Model file for the job. Use its own axes, mm. A direction names the side the tool comes from. Give positions to 0.01 mm unless a question says otherwise; leave off trailing zeros. Loops run counter-clockwise (first coordinate to the right, second up) from the corner with the lowest first, then second, coordinate; pieces in that order, holes last. Notation, with made-up numbers: (45.25, 70) - (67.25, 70) arc R15 cw to (67.25, 97) - close; hole circle Ø2 at (48, 56.25). An arc over 180 degrees is marked (long way). Answer as CSV lines item,"result". Start each with the question number.
Item 1: Drill centre lines: L1, parallel to Y at x = 5.5, z = 10.75; L2, parallel to Y at x = -53.45, z = 8.5; L3, parallel to X at y = -7, z = 13.5. Where is each one in solid material? Low to high. Write a range as from..to.
Item 2: Pull direction Z, two halves, no side cores. Call faces 1 (the flat face through (54, -5, 8)), 2 (the flat face through (-1, 5, 2.5)), 3 (the flat face through (-1, 12, 0)): pulls with the +Z half, pulls with the -Z half, needs draft (parallel to the pull), parting line crosses it, or undercut.
Item 3: Saw through at B-B on x = -45. Give the cut face in (y, z), plus the area to 3 significant figures.
Item 4: Saw through at A-A on y = -5. Give the cut face in (x, z).
Item 5: Tool access for faces 4 (the flat face through (39, 29.41, 1)), 5 (the cylindrical face through (54.014, 3.6, 10.325)), 6 (the flat face through (-1, -5, 2.5)), 7 (the flat face through (-39, 29.41, 1)), 8 (the cylindrical face through (53.493, -6.4, 6.675)): list every direction of +Z, -Z, +X, -X, +Y, -Y with a clear straight run to the whole face (end or side of a thin tool).
Item 6: Pin check, flat tips, straight feed: pin 1 (6 mm diameter, centred on x = 8, z = 9.5, fed in from -Y); pin 2 (1.5 mm diameter, centred on y = 11.5, z = 8.5, fed in from +X); pin 3 (4 mm diameter, centred on y = -5, z = 8.5, fed in from -X). Stop position of each tip, or through.
Item 7: Saw through at D-D on y = 32. Give the cut face in (x, z).
Item 8: Saw through at C-C on z = 13. Give the cut face in (x, y).
from build123d import *

# Parameters (mm, degrees)
SKETCH1_W           = 150
SKETCH1_H           = 41.41
BOSS_EXTRUDE1_DEPTH = 2.5
SKETCH5_W           = 110
SKETCH5_H           = 22
BOSS_EXTRUDE3_DEPTH = 12
SKETCH6_W           = 106
SKETCH6_H           = 8
CUT_EXTRUDE3_DEPTH  = 12
SKETCH7_R           = 2.3
CUT_EXTRUDE4_DEPTH  = 109
SKETCH8_R           = 2.3
CUT_EXTRUDE5_DEPTH  = 109
SKETCH9_W           = 7.040043687
SKETCH9_H           = 2.5
BOSS_EXTRUDE4_DEPTH = 20


with BuildPart() as part:
    # Sketch1 → Boss-Extrude1 (new body)
    with BuildSketch(Plane.XY):
        with Locations((0, 8.705)):
            Rectangle(SKETCH1_W, SKETCH1_H)
    extrude(amount=BOSS_EXTRUDE1_DEPTH)

    # Sketch5 → Boss-Extrude3 (add)
    with BuildSketch(Plane.XY.offset(2.5)):
        Rectangle(SKETCH5_W, SKETCH5_H)
    extrude(amount=BOSS_EXTRUDE3_DEPTH)

    # Sketch6 → Cut-Extrude3 (cut)
    with BuildSketch(Plane.XY.offset(2.5)):
        with Locations((0, 5)):
            Rectangle(SKETCH6_W, SKETCH6_H)
        with Locations((0, -5)):
            Rectangle(SKETCH6_W, SKETCH6_H)
    extrude(amount=CUT_EXTRUDE3_DEPTH, mode=Mode.SUBTRACT)

    # Sketch7 → Cut-Extrude4 (cut)
    with BuildSketch(Plane.ZY.offset(55)):
        with Locations((8.5, -5)):
            Circle(SKETCH7_R)
    extrude(amount=-CUT_EXTRUDE4_DEPTH, mode=Mode.SUBTRACT)

    # Sketch8 → Cut-Extrude5 (cut)
    with BuildSketch(Plane(origin=(55, 0, 0), x_dir=(0, 0, -1), z_dir=(1, 0, 0))):
        with Locations((-8.5, 5)):
            Circle(SKETCH8_R)
    extrude(amount=-CUT_EXTRUDE5_DEPTH, mode=Mode.SUBTRACT)

    # Sketch9 → Boss-Extrude4 (add)
    with BuildSketch(Plane(origin=(0, 29.41, 0), x_dir=(1, 0, 0), z_dir=(0, 1, 0))):
        with Locations((0.645201015, -1.25)):
            Rectangle(SKETCH9_W, SKETCH9_H)
    extrude(amount=BOSS_EXTRUDE4_DEPTH)


solid = part.part
Responses:
1,L1,"-11..-9, -1..1, 9..11"
1,L2,"-11..-7.3, -2.7..2.7, 7.3..11"
1,L3,"-55..-53, 53..55"
2,face 1,"undercut"
2,face 2,"pulls with the +Z half"
2,face 3,"pulls with the -Z half"
3,outline,"(-12, 0) - (29.41, 0) - (29.41, 2.5) - (11, 2.5) - (11, 14.5) - (9, 14.5) - (9, 2.5) - (1, 2.5) - (1, 14.5) - (-1, 14.5) - (-1, 2.5) - (-9, 2.5) - (-9, 14.5) - (-11, 14.5) - (-11, 2.5) - (-12, 2.5) - close"
3,area,"176 mm2"
4,outline,"(-75, 0) - (75, 0) - (75, 2.5) - (55, 2.5) - (55, 14.5) - (53, 14.5) - (53, 10.8) - (54, 10.8) - (54, 6.2) - (53, 6.2) - (53, 2.5) - (-53, 2.5) - (-53, 6.2) - (-55, 6.2) - (-55, 2.5) - (-75, 2.5) - close; (-55, 10.8) - (-53, 10.8) - (-53, 14.5) - (-55, 14.5) - close"
5,face 4,"+Z, -Z, +X, +Y"
5,face 5,"+X"
5,face 6,"+Z"
5,face 7,"+Z, -Z, -X, +Y"
5,face 8,"-X"
6,pin 1,"y = -11"
6,pin 2,"x = 55"
6,pin 3,"x = 54"
7,outline,"(-2.87, 0) - (4.17, 0) - (4.17, 2.5) - (-2.87, 2.5) - close"
8,outline,"(-55, -11) - (55, -11) - (55, 11) - (-55, 11) - close; hole (-53, -9) - (53, -9) - (53, -1) - (-53, -1) - close; hole (-53, 1) - (53, 1) - (53, 9) - (-53, 9) - close"
